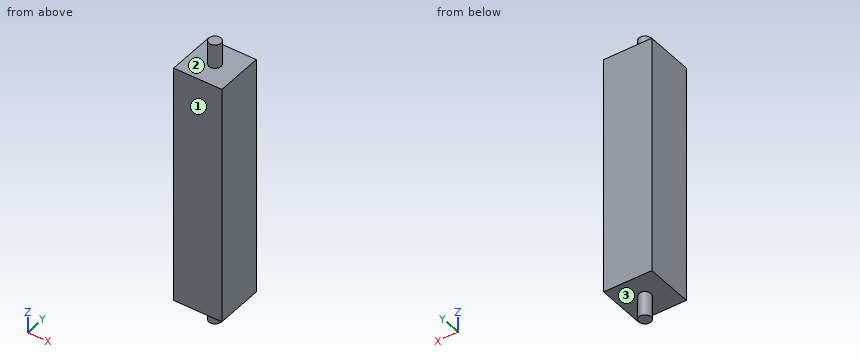
```python
from build123d import *

# Parameters (mm, degrees)
SKETCH_W     = 40
SKETCH_H     = 200
PAD_DEPTH    = 40
SKETCH001_R  = 5
PAD001_DEPTH = 20
PAD002_DEPTH = 220


with BuildPart() as part:
    # Sketch → Pad (new body)
    with BuildSketch(Plane.XZ):
        with Locations((20, 100)):
            Rectangle(SKETCH_W, SKETCH_H)
    extrude(amount=PAD_DEPTH)

    # Sketch001 → Pad001 (join)
    with BuildSketch(Plane.XY):
        with Locations((20, -20)):
            Circle(SKETCH001_R)
    extrude(amount=-PAD001_DEPTH)

    # Sketch001 → Pad002 (join)
    with BuildSketch(Plane.XY):
        with Locations((20, -20)):
            Circle(SKETCH001_R)
    extrude(amount=PAD002_DEPTH)


solid = part.part
```
Here's how the part is built. I have some questions about the finished solid (model axes, mm). Face numbers are marked on the shaded views. A direction names the side the tool comes from. Round coordinates to 2 decimals unless told otherwise and drop trailing zeros. Order: outer loops, then holes, each group sorted by start corner. A loop starts at its lowest first (then second) coordinate and runs counter-clockwise, first axis right, second up. Notation, with made-up numbers: M 54.5,8 L 76.5,8 A15 ccw 76.5,27 Z; hole C -37.75,21 d10. An arc over 180 degrees is marked long. Answer in a Markdown table with one row per item.
Item 1: Imagine slicing it at D-D, the plane x = 29. Write out the boundary of the cut face in (y, z).
A:
| item | result |
|---|---|
| outline | M -40,0 L 0,0 L 0,200 L -40,200 Z |
Item 2: Imagine slicing it at B-B, the plane x = 20. Write out the boundary of the cut face in (y, z), and give its area (3 significant figures).
A:
| item | result |
|---|---|
| outline | M -40,0 L -25,0 L -25,-20 L -15,-20 L -15,0 L 0,0 L 0,200 L -15,200 L -15,220 L -25,220 L -25,200 L -40,200 Z |
| area | 8,400 mm2 |
Item 3: If I drill on L1, parallel to Z at x = 13.5, y = -28; L2, parallel to X at y = -24, z = 207.5, over which ranges is the centre line in solid material (lowest first)? Write a range as from..to.
A:
| item | result |
|---|---|
| L1 | z = 0..200 |
| L2 | x = 17..23 |
Item 4: Imagine slicing it at A-A, the plane y = -20. Write out the boundary of the cut face in (x, z), and give its area (3 significant figures).
A:
| item | result |
|---|---|
| outline | M 0,0 L 15,0 L 15,-20 L 25,-20 L 25,0 L 40,0 L 40,200 L 25,200 L 25,220 L 15,220 L 15,200 L 0,200 Z |
| area | 8,400 mm2 |
Item 5: For the marked faces 1, 2 and 3, which set-ups out of +Z, -Z, +X, -X, +Y, -Y let a thin tool reach every point of the face, with its end or its side?
A:
| item | result |
|---|---|
| face 1 | +Z, -Z, +X, -X, -Y |
| face 2 | +Z |
| face 3 | -Z |
Item 6: Imagine slicing it at C-C, the plane y = -9. Write out the boundary of the cut face in (x, z).
A:
| item | result |
|---|---|
| outline | M 0,0 L 40,0 L 40,200 L 0,200 Z |
Item 7: I'm going to push flat-ended pins straight in: pin 1 (10 mm diameter, centred on x = 6, y = -26.5, fed in from -Z); pin 2 (5 mm diameter, centred on y = -34, z = 65.5, fed in from -X); pin 3 (10 mm diameter, centred on x = 26.5, y = -9.5, fed in from +Z). Where does each tip first touch, or does it pass through?
A:
| item | result |
|---|---|
| pin 1 | stops at z = 0 |
| pin 2 | stops at x = 0 |
| pin 3 | stops at z = 200 |
